Autodesk Inventor part; units mm, degrees
ref_plane "YZ Plane" through (0, 0, 0) normal (1, 0, 0) x (0, 1, 0)
ref_plane "XZ Plane" through (0, 0, 0) normal (0, 1, 0) x (-1, 0, 0)
ref_plane "XY Plane" through (0, 0, 0) normal (0, 0, 1) x (1, 0, 0)
sketch "Skizze1" plane through (0, 0, 0) normal (1, 0, 0) x (0, 1, 0)
  line L0 (0, 17.7) -> (0, -2.95) construction
  line L1 (-59.5, 0) -> (59.5, 0)
  line L2 (42.5, 8) -> (42.5, 0)
  line L3 (42.5, 8) -> (27.5, 8)
  line L4 (27.5, 8) -> (27.5, 10)
  line L5 (27.5, 10) -> (-11.1, 10)
  line L6 (-11.1, 10) -> (-11.1, 14.75)
  line L7 (-11.1, 14.75) -> (-27.5, 14.75)
  line L8 (-27.5, 14.75) -> (-27.5, 8)
  line L9 (-27.5, 8) -> (-42.5, 8)
  line L10 (-42.5, 8) -> (-42.5, 0)
  line L11 (-11.1, 14.75) -> (11.1, 14.75) construction
  line L12 (11.1, 14.75) -> (11.1, 10) construction
  line L13 (-42.5, 0) -> (42.5, 0)
  point P0 (0, 0)
  dimension "d0" = 16
  dimension "d1" = 15
  dimension "d2" = 22.2
  dimension "d3" = 55
  dimension "d4" = 20
  dimension "d5" = 29.5
revolve "Grundkörper" add sketch "Skizze1" angle 360 about axis through (0, 0, 0) along (0, 1, 0)
sketch "Skizze2" plane through (0, 0, 0) normal (1, 0, 0) x (0, 1, 0)
  line L0 (-9.1, 0) -> (33.6, 0) construction
  line L1 (-11.1, -14.75) -> (-11.1, 14.75) construction
  line L2 (-11.1, 10) -> (27.5, 10)
  line L3 (-11.1, 10) -> (-11.1, 14.75)
  line L4 (-11.1, 14.75) -> (11.1, 14.75)
  line L5 (11.1, 14.75) -> (11.1, 10)
  line L6 (11.1, 10) -> (-11.1, 10)
  line L7 (0, 20.65) -> (0, -20.65) construction
  line L8 (11.1, 10) -> (11.1, 9.5)
  line L9 (11.1, 9.5) -> (12.4, 9.5)
  line L10 (12.4, 9.5) -> (12.4, 10)
  line L11 (11.1, 10) -> (12.4, 10)
  point P0 (0, 0)
  dimension "d15" = 1.3
  dimension "d16" = 19
revolve "Nut_Sicherungsring_DIN471-20x1,2" cut sketch "Skizze2" angle 360 about axis through (0, 0, 0) along (0, 1, 0) contours L2 L10 L9 L8
chamfer "FaseAllgemein" distance 1 angle 45 3 edges at (0, -42.5, -8) (0, 42.5, -8) (0, -27.5, -14.75)
chamfer "FaseLager" distance 0.5 angle 45 1 edges at (0, -11.1, -14.75)
properties part number "200-40-BOGIE-CONNECTOR-05" material "Aluminium 6061"
Design review of the part built by this model. Coordinates are the model's own, in mm. A direction names the side the tool comes from. Round coordinates to 2 decimals unless told otherwise and drop trailing zeros. Write each loop counter-clockwise with the first axis right and the second up, starting at its lowest first coordinate (ties: lowest second). Pieces come first, ordered by that corner, then holes. Notation, with made-up numbers: (73.25, 24) -> (122.25, 24) arc R33 ccw to (122.25, 60) -> close; hole circle Ø11 at (-2, 79). An arc over 180 degrees is marked (long way). Answer in a Markdown table with one row per item.
Q1. Take a section at C-C, the plane y = 8. State the section outline as (x, z) points, then the cut area to 3 significant figures.
The answers:
| item | result |
|---|---|
| outline | circle Ø20 at (0, 0) |
| area | 314 mm² |
Q2. For faces 4 (the face through (7.81, 34.4, -1.73)), 5 (the face through (0, -42.5, 0)), 6 (the face through (-4.43, -19.15, 14.07)), 7 (the face through (-6, -27.5, 6)), 8 (the face through (-8.43, 11.76, 4.38)), list the 3-axis set-ups (+Z, -Z, +X, -X, +Y, -Y) from which the entire face can be reached by the end or side of a thin tool; tool diameter is ignored.
The answers:
| item | result |
|---|---|
| face 4 | +Y |
| face 5 | +Z, -Z, +X, -X, -Y |
| face 6 | +Y, -Y |
| face 7 | -Y |
| face 8 | none |
Q3. Clearance check with flat-ended pins moving along their axes: pin 1 Ø4 at (x, z) = (-6, 8.5) entering from -Y; pin 2 Ø1.5 at (x, y) = (4, 4) entering from -Z; pin 3 Ø10 at (x, y) = (-9, 20.5) entering from +Z; pin 4 Ø4 at (x, z) = (-2.5, -7) entering from -Y. State where each tip first meets the part, or that it passes through.
The answers:
| item | result |
|---|---|
| pin 1 | y = -27.5 |
| pin 2 | z = -9.46 |
| pin 3 | z = 9.17 |
| pin 4 | y = -42.5 |
Q4. Draft analysis for pull direction Y (two halves, no side actions). For faces 1 (the face through (-4, 11.1, 9)), 2 (the face through (0, 42.5, 0)), 3 (the face through (7.81, -34.6, -1.73)), state which applies: +Y half, -Y half, draft (parallel to the pull), parting line (faces both ways), or undercut.
The answers:
| item | result |
|---|---|
| face 1 | undercut |
| face 2 | +Y half |
| face 3 | draft |
Q5. To check wall thickness, follow L1, parallel to Y at x = -9.25, z = -8.75; L2, parallel to Y at x = -8, z = -5.25; L3, parallel to Y at x = 5.75, z = 6. State the ranges of each line that lie inside material, in increasing order. Write a range as [from, to].
The answers:
| item | result |
|---|---|
| L1 | [-27.5, -11.1] |
| L2 | [-27.5, 11.1], [12.4, 27.5] |
| L3 | [-27.5, 27.5] |
